Model file for the job. Use its own axes, mm. A direction names the side the tool comes from. Round coordinates to 2 decimals unless told otherwise and drop trailing zeros. Loops run counter-clockwise (first coordinate to the right, second up) from the corner with the lowest first, then second, coordinate; pieces in that order, holes last. Notation, with made-up numbers: (43, 7.5) - (89, 7.5) arc R17 cw to (89, 39.5) - close; hole circle Ø8 at (49, 17). An arc over 180 degrees is marked (long way). Answer as a JSON object with one key per item and string values.
from build123d import *

# Parameters (mm, degrees)
SKETCH1_W           = 241.3
SKETCH1_H           = 50.8
BOSS_EXTRUDE1_DEPTH = 19.06
SKETCH3_R           = 4
CUT_EXTRUDE1_DEPTH  = 125.759232524
CUT_EXTRUDE2_DEPTH  = 125.759232524
SKETCH11_R          = 15.09
CUT_EXTRUDE3_DEPTH  = 125.759232524
BOSS_EXTRUDE2_DEPTH = 19.06
CUT_EXTRUDE4_DEPTH  = 125.759232524


with BuildPart() as part:
    # Sketch1 → Boss-Extrude1 (new body)
    with BuildSketch(Plane.XY):
        Rectangle(SKETCH1_W, SKETCH1_H)
    extrude(amount=BOSS_EXTRUDE1_DEPTH)

    # Sketch3 → Cut-Extrude1 (cut, through all)
    with BuildSketch(Plane.XY.offset(19.06)):
        with Locations((-107.95, 0)):
            Circle(SKETCH3_R)
    extrude(amount=-CUT_EXTRUDE1_DEPTH, mode=Mode.SUBTRACT)

    # Sketch5 → Cut-Extrude2 (cut, through all)
    with BuildSketch(Plane.XY.offset(19.06)):
        with BuildLine():
            ThreePointArc((67.637087091, -25.4), (97.003321964, -2.984354021), (120.65, 25.4))
            Line((120.65, 25.4), (120.65, -25.4))
            Line((120.65, -25.4), (67.637087091, -25.4))
        make_face()
        with BuildLine():
            Line((-62.046109456, -25.4), (-107.95, -6.35))
            ThreePointArc((-107.95, -6.35), (-114.3, 0), (-107.95, 6.35))
            Line((-107.95, 6.35), (-65.239311186, 25.4))
            Line((-65.239311186, 25.4), (-120.65, 25.4))
            Line((-120.65, 25.4), (-120.65, -25.4))
            Line((-120.65, -25.4), (-62.046109456, -25.4))
        make_face()
    extrude(amount=-CUT_EXTRUDE2_DEPTH, mode=Mode.SUBTRACT)

    # Sketch11 → Cut-Extrude3 (cut, through all)
    with BuildSketch(Plane(origin=(0, 0, 0), x_dir=(-1, 0, 0), z_dir=(0, 0, -1))):
        with Locations((-70.2, 0)):
            Circle(SKETCH11_R)
    extrude(amount=-CUT_EXTRUDE3_DEPTH, mode=Mode.SUBTRACT)

    # Sketch12 → Boss-Extrude2 (add)
    with BuildSketch(Plane(origin=(0, 0, 0), x_dir=(-1, 0, 0), z_dir=(0, 0, -1))):
        Polygon((86.939525855, -21.602548055), (79.526368634, -18.145736072), (90.717044303, -13.501633601), align=None)
    extrude(amount=-BOSS_EXTRUDE2_DEPTH)

    # Sketch13 → Cut-Extrude4 (cut, through all)
    with BuildSketch(Plane(origin=(0, 0, 0), x_dir=(-1, 0, 0), z_dir=(0, 0, -1))):
        with BuildLine():
            Line((-91.17795532, 15.24), (-100.287694386, 15.24))
            ThreePointArc((-100.287694386, 15.24), (-97.460762969, 12.040493243), (-94.546748719, 8.920091718))
            ThreePointArc((-94.546748719, 8.920091718), (-93.081597611, 12.196913552), (-91.17795532, 15.24))
        make_face()
        Polygon((13.984519796, -15.24), (60.021626843, -15.24), (79.764838161, -7.046616582), (83.177072141, -5.630547997), (97.003760461, 0.107493144), (63.076212362, 15.24), (13.984519796, 15.24), align=None)
        with BuildLine():
            Line((2.07417074, -15.24), (2.07417074, 15.24))
            Line((2.07417074, 15.24), (-49.22204468, 15.24))
            ThreePointArc((-49.22204468, 15.24), (-44.27063037, 0), (-49.22204468, -15.24))
            Line((-49.22204468, -15.24), (2.07417074, -15.24))
        make_face()
    extrude(amount=-CUT_EXTRUDE4_DEPTH, mode=Mode.SUBTRACT)


solid = part.part
1) Two-plate mould, pull along X, no slides. Class faces 4 (the flat face through (-86.894, 15.742, 9.663)), 5 (the cylindrical face through (96.63, -3.34, 9.66)), 6 (the cylindrical face through (-111.946, 0.176, 9.663)): pulls with the +X half, pulls with the -X half, needs draft (parallel to the pull), parting line crosses it, or undercut.
Values follow:
{"face 4": "pulls with the -X half", "face 5": "pulls with the +X half", "face 6": "undercut"}
2) Tool access for faces 1 (the flat face through (-83.285, -19.898, 9.397)), 2 (the flat face through (2, 17, 0)), 3 (the flat face through (-13.985, 0, 9)): list every direction of +Z, -Z, +X, -X, +Y, -Y with a clear straight run to the whole face (end or side of a thin tool).
Values follow:
{"face 1": "+Z, -Z, -Y", "face 2": "-Z, +X, -X, +Y, -Y", "face 3": "+Z, -Z"}
3) Probe probe 1 along Y at (x, z) = (-34, 16.25); probe 2 along X at (y, z) = (4.5, 17.75); probe 3 along Y at (x, z) = (-107.95, 7.75). List the from-to ranges inside material, lowest first.
Values follow:
{"probe 1": "-25.4 to -15.24, 15.24 to 25.4", "probe 2": "-112.43 to -87.16, -13.98 to -2.07, 44.66 to 55.8, 84.6 to 104.33", "probe 3": "-6.35 to -4, 4 to 6.35"}
4) Slice it at C-C on z = 12.5. List the corners of the cut face in (x, y).
Values follow:
{"outline": "(-107.95, -6.35) - (-90.72, -13.5) - (-86.94, -21.6) - (-79.53, -18.15) - (-62.05, -25.4) - (67.64, -25.4) arc R165.1 ccw to (120.65, 25.4) - (-65.24, 25.4) - (-107.95, 6.35) arc R6.35 ccw to start; hole circle Ø8 at (-107.95, 0); hole (-97, 0.11) - (-60.02, -15.24) - (-13.98, -15.24) - (-13.98, 15.24) - (-63.08, 15.24) - close; hole (-2.07, -15.24) - (49.22, -15.24) arc R25.93 cw to (49.22, 15.24) - (-2.07, 15.24) - close; hole circle Ø30.18 at (70.2, 0); hole (91.18, 15.24) arc R25.93 cw to (94.55, 8.92) arc R154.94 ccw to (100.29, 15.24) - close"}
5) Drop flat-ended pins along their axis: P1, Ø6, axis at x = 1, y = -11.5, coming from the +Z side; P2, Ø2, axis at y = 1.5, z = 9.5, coming from the -X side; P3, Ø2.5, axis at x = 94.5, z = 10, coming from the -Y side; P4, Ø2, axis at x = 91, z = 6.5, coming from the -Y side. Give the stop position or say it passes through.
Values follow:
{"P1": "through", "P2": "x = -114.28", "P3": "y = -6.47", "P4": "y = -9.32"}
6) Slice it at B-B on y = 13. List the corners of the cut face in (x, z), then the cut area to 3 significant figures.
Values follow:
{"outline": "(-93.04, 0) - (-68.1, 0) - (-68.1, 19.06) - (-93.04, 19.06) - close; (-13.98, 0) - (-2.07, 0) - (-2.07, 19.06) - (-13.98, 19.06) - close; (47.76, 0) - (62.54, 0) - (62.54, 19.06) - (47.76, 19.06) - close; (77.86, 0) - (92.64, 0) - (92.64, 19.06) - (77.86, 19.06) - close; (98.33, 0) - (111.63, 0) - (111.63, 19.06) - (98.33, 19.06) - close", "area": "1,520 mm²"}
7) Slice it at A-A on x = -28. List the corners of the cut face in (y, z).
Values follow:
{"outline": "(-25.4, 0) - (-15.24, 0) - (-15.24, 19.06) - (-25.4, 19.06) - close; (15.24, 0) - (25.4, 0) - (25.4, 19.06) - (15.24, 19.06) - close"}
8) Slice it at D-D on y = -10. List the corners of the cut face in (x, z), then the cut area to 3 significant figures.
Values follow:
{"outline": "(-99.15, 0) - (-72.65, 0) - (-72.65, 19.06) - (-99.15, 19.06) - close; (-13.98, 0) - (-2.07, 0) - (-2.07, 19.06) - (-13.98, 19.06) - close; (46.28, 0) - (58.9, 0) - (58.9, 19.06) - (46.28, 19.06) - close; (81.5, 0) - (89.2, 0) - (89.2, 19.06) - (81.5, 19.06) - close", "area": "1,120 mm²"}
